Can you work these out from the drawing? Everything is in mm from the part's minimum corner. Round coordinates to 2 decimals unless told otherwise and drop trailing zeros. Loops run counter-clockwise (first coordinate to the right, second up) from the corner with the lowest first, then second, coordinate; pieces in that order, holes last. Notation, with made-up numbers: M 88,-26.5 L 114,-26.5 A32 cw 114,2.5 Z; hole C 70,21 d4. An arc over 180 degrees is marked long. Answer in a Markdown table with one row per item.
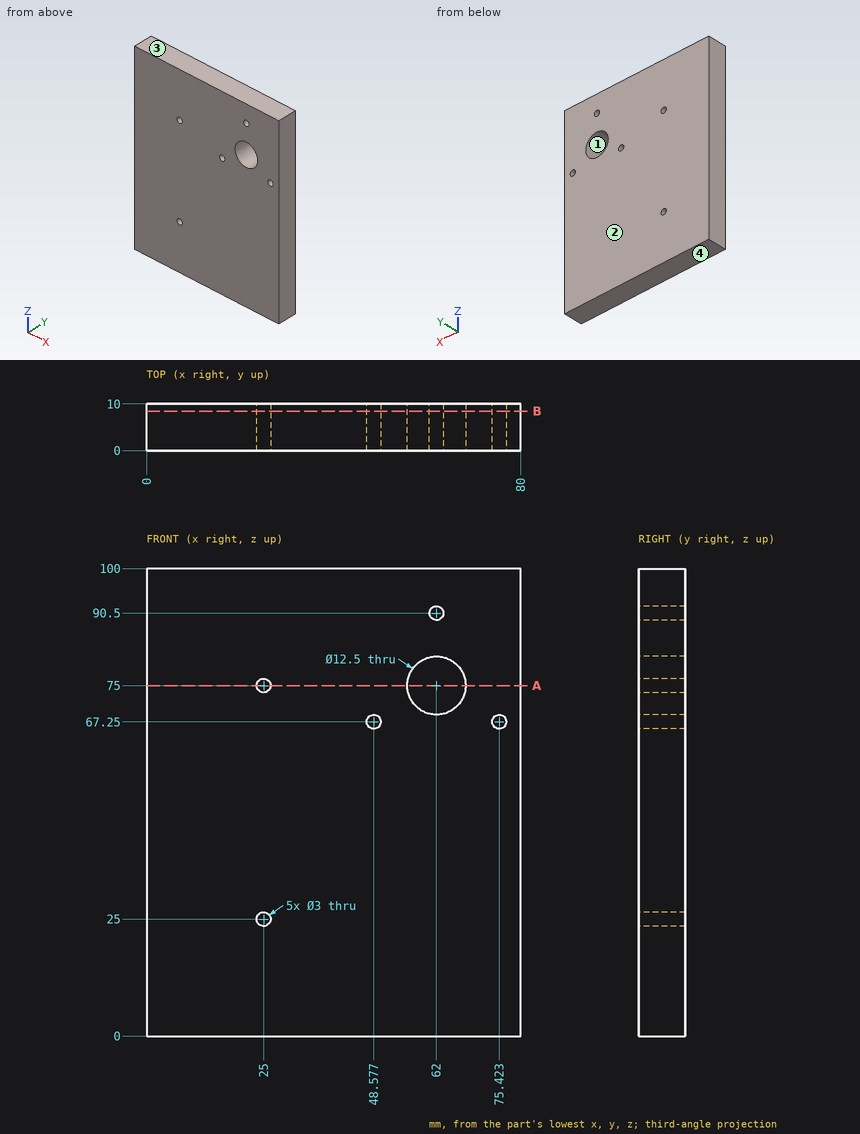
1) I need wall thicknesses on line 1 (Z direction, x = 62, y = 2.5); line 2 (Z direction, x = 25, y = 3.25); line 3 (X direction, y = 7.75, z = 67.25). Which ranges of each line are inside material? Lowest first, please.
Computed:
| item | result |
|---|---|
| line 1 | z = 0 to 68.75, 81.25 to 89, 92 to 100 |
| line 2 | z = 0 to 23.5, 26.5 to 73.5, 76.5 to 100 |
| line 3 | x = 0 to 47.08, 50.08 to 73.92, 76.92 to 80 |
2) Will this pin go through, and if not, where does the flat tip stop? P1, Ø2.5, axis at x = 25, z = 25, coming from the +Y side.
Computed:
| item | result |
|---|---|
| P1 | passes through |
3) If we mould it in two halves opening along Z, with no side actions, what happens to the marked faces 1, 2, 3 and 4? For each: released by +Z, released by -Z, zero draft, split by the parting line, or undercut.
Computed:
| item | result |
|---|---|
| face 1 | undercut |
| face 2 | zero draft |
| face 3 | released by +Z |
| face 4 | released by -Z |
4) I want a section at B-B, the plane y = 8.5. Please give me the cut outline in (x, z), plus the area to 3 significant figures.
Computed:
| item | result |
|---|---|
| outline | M 0,0 L 80,0 L 80,100 L 0,100 Z; hole C 25,25 d3; hole C 25,75 d3; hole C 48.58,67.25 d3; hole C 62,75 d12.5; hole C 62,90.5 d3; hole C 75.42,67.25 d3 |
| area | 7,840 mm² |
5) I want a section at A-A, the plane z = 75. Please give me the cut outline in (x, y).
Computed:
| item | result |
|---|---|
| outline | M 0,0 L 23.5,0 L 23.5,10 L 0,10 Z; M 26.5,0 L 55.75,0 L 55.75,10 L 26.5,10 Z; M 68.25,0 L 80,0 L 80,10 L 68.25,10 Z |
